Autodesk Fusion 360 part; units mm, degrees
sketch "Sketch1" plane through (0, 0, 0) normal (0, 0, 1) x (1, 0, 0)
  line L0 (21, -26) -> (-21, -26) construction
  line L1 (-21, -26) -> (-21, 26) construction
  line L2 (-21, 26) -> (21, 26) construction
  line L3 (21, 26) -> (21, -26) construction
  line L4 (21, -26) -> (-21, 26) construction
  line L5 (-21, -26) -> (21, 26) construction
  circle A0 centre (-21, 26) radius 1.4
  circle A1 centre (21, 26) radius 1.4
  circle A2 centre (-21, -26) radius 1.4
  circle A3 centre (21, -26) radius 1.4
  line L6 (10, 45) -> (-10, 45) construction
  line L7 (-10, 45) -> (-10, -45) construction
  line L8 (-10, -45) -> (10, -45) construction
  line L9 (10, -45) -> (10, 45) construction
  line L10 (10, 45) -> (-10, -45) construction
  line L11 (-10, 45) -> (10, -45) construction
  circle A4 centre (-10, 45) radius 1.625
  circle A5 centre (10, 45) radius 1.625
  circle A6 centre (21, -26) radius 4
  circle A7 centre (-21, -26) radius 4
  circle A8 centre (-21, 26) radius 4
  circle A9 centre (21, 26) radius 4
  circle A10 centre (-10, 45) radius 4
  circle A11 centre (10, 45) radius 4
  line L12 (25, -26) -> (-25, -26) construction
  line L13 (-25, -26) -> (-25, 26) construction
  line L14 (-25, 26) -> (25, 26) construction
  line L15 (25, 26) -> (25, -26) construction
  line L16 (25, -26) -> (-25, 26) construction
  line L17 (-25, -26) -> (25, 26) construction
  line L18 (21, -30) -> (-21, -30) construction
  line L19 (-21, -30) -> (-21, 30) construction
  line L20 (-21, 30) -> (21, 30) construction
  line L21 (21, 30) -> (21, -30) construction
  line L22 (21, -30) -> (-21, 30) construction
  line L23 (-21, -30) -> (21, 30) construction
  line L24 (25, -30) -> (-25, -30)
  line L25 (-25, -30) -> (-25, 30)
  line L26 (-25, 30) -> (25, 30)
  line L27 (25, 30) -> (25, -30)
  line L28 (-21, 26) -> (21, 26)
  line L29 (21, 26) -> (21, 49.335)
  line L30 (21, 49.335) -> (-21, 49.335)
  line L31 (-21, 49.335) -> (-21, 26)
  dimension "d1" = 52
  dimension "d2" = 42
  dimension "d3" = 2.8
  dimension "d4" = 2.8
  dimension "d5" = 2.8
  dimension "d6" = 2.8
  dimension "d7" = 90
  dimension "d8" = 20
  dimension "d9" = 3.25
  dimension "d10" = 3.25
  dimension "d11" = 8
  dimension "d12" = 8
  dimension "d13" = 8
  dimension "d14" = 8
  dimension "d15" = 8
  dimension "d16" = 8
  dimension "d17" = 60
  dimension "d18" = 50
extrude "Extrude1" add sketch "Sketch1" along normal blind 3 contours A6 A7 A8 A9 L24 L25 L27 L28 | A8 A9 L26 L28 | A8 L25 L26 | A9 L26 L27 | A7 L24 L25 | A6 L24 L27
extrude "Extrude2" add sketch "Sketch1" along normal blind 10 contours A0 A8 L28 L31 | A0 A8 L28 L31 | A1 A9 L28 L29 | A1 A9 L28 L29 | A7 | A6
sketch "Sketch2" plane through (0, 0, 3) normal (0, 0, 1) x (-1, 0, 0)
  line L0 (25, -26) -> (25, 26)
  line L1 (21, 30) -> (-21, 30)
  line L2 (-25, 26) -> (-25, -26)
  circle A0 centre (0, -15) radius 1.75
  circle A1 centre (0.0425, 15) radius 1.75
  line L3 (-21, -30) -> (21, -30)
  circle A2 centre (0, 0) radius 9
  circle A3 centre (15, -15) radius 6
  circle A4 centre (-15, -15) radius 6
  circle A5 centre (-15, 15) radius 6
  circle A6 centre (15, 15) radius 6
  arc A7 (-21, -30) -> (-25, -26) centre (-21, -26) ccw
  arc A8 (25, -26) -> (21, -30) centre (21, -26) ccw
  arc A9 (21, 30) -> (25, 26) centre (21, 26) ccw
  arc A10 (-25, 26) -> (-21, 30) centre (-21, 26) ccw
  dimension "d23" = 3.5
  dimension "d24" = 3.5
  dimension "d25" = 15
  dimension "d26" = 15
  dimension "d29" = 18
  dimension "d30" = 12
  dimension "d31" = 12
  dimension "d32" = 12
  dimension "d33" = 12
  dimension "d34" = 10
  dimension "d35" = 10
  dimension "d36" = 10
  dimension "d37" = 10
  dimension "d38" = 15
  dimension "d39" = 15
  dimension "d40" = 15
  dimension "d41" = 15
extrude "Extrude3" cut sketch "Sketch2" against normal blind 9 contours A0 | A1 | A2 | A3 | A4 | A5 | A6
equation "d35 = d34"
equation "d36 = d34"
equation "d37 = d34"
equation "d39 = d38"
equation "d40 = d38"
equation "d41 = d38"
Input: part model. Units: mm. Frame: model coordinates. A direction names the side the tool comes from. Coordinates: 2 decimals unless noted, no trailing zeros. Loops run counter-clockwise (first coordinate to the right, second up) from the corner with the lowest first, then second, coordinate; pieces in that order, holes last. Notation, with made-up numbers: M 72,-8.75 L 91,-8.75 A6 ccw 91,1.25 Z; hole C 48.25,56.25 d11. An arc over 180 degrees is marked long. One line per item, written item: value.
(1) Reachability of faces 1 (the flat face through (-24, -29, 3)), 2 (the cylindrical face through (22.29, -25.46, 4.93)), 3 (the cylindrical face through (18.05, -28.7, 6.45)), 4 (the flat face through (24, 29, 3)), 5 (the flat face through (-24, 29, 3)) from +Z, -Z, +X, -X, +Y, -Y: full face, straight path, thin tool, end or side. Return the list, or none.
Filled in:
face 1: +Z, -X, -Y
face 2: +Z, -Z
face 3: +Z
face 4: +Z, +X, +Y
face 5: +Z, -X, +Y
(2) Section B-B (y = -15). Output: boundary loops of the cut face in (x, z).
Filled in:
outline: M -25,0 L -21,0 L -21,3 L -25,3 Z; M -9,0 L -1.79,0 L -1.79,3 L -9,3 Z; M 1.71,0 L 9,0 L 9,3 L 1.71,3 Z; M 21,0 L 25,0 L 25,3 L 21,3 Z
(3) Section A-A (z = 4.25). Output: boundary loops of the cut face in (x, y), and give its area (3 significant figures).
Filled in:
outline: C -21,-26 d8; C -21,26 d8; C 21,-26 d8; C 21,26 d8; hole C -21,-26 d2.8; hole C -21,26 d2.8; hole C 21,-26 d2.8; hole C 21,26 d2.8
area: 176 mm^2
(4) Section D-D (x = -4.5). Output: boundary loops of the cut face in (y, z).
Filled in:
outline: M -30,0 L -7.79,0 L -7.79,3 L -30,3 Z; M 7.79,0 L 30,0 L 30,3 L 7.79,3 Z
(5) Pin query (flat end, axial travel): pin 1 (10 mm diameter, centred on x = -2, y = 1, fed in from +Z). Return the tip coordinate at first contact, or that it passes through.
Filled in:
pin 1: through
(6) Pull-direction query (X, two-part tool) for faces 6 (the flat face through (23, -26, 10)), 7 (the flat face through (-6, 7, 3)), 8 (the flat face through (-25, 0, 1)); classes: +X half, -X half, draft (parallel to the pull), parting line (faces both ways), or undercut.
Filled in:
face 6: draft
face 7: undercut
face 8: -X half
(7) Line query: line 1 along X through (y, z) = (-15, 1.8); line 2 along X through (y, z) = (26, 7); line 3 along Y through (x, z) = (-21, 4). Output: solid intervals per line, ascending. Write a range as from..to.
Filled in:
line 1: -25..-21, -9..-1.79, 1.71..9, 21..25
line 2: -25..-22.4, -19.6..-17, 17..19.6, 22.4..25
line 3: -30..-27.4, -24.6..-22, 22..24.6, 27.4..30
(8) Section C-C (x = -15). Output: boundary loops of the cut face in (y, z).
Filled in:
outline: M -30,0 L -21,0 L -21,3 L -30,3 Z; M -9,0 L 9,0 L 9,3 L -9,3 Z; M 21,0 L 30,0 L 30,3 L 21,3 Z
